The model under review builds one solid part; all positions refer to its coordinate system, in mm. Face numbers are marked on the shaded views. A direction names the side the tool comes from. Round coordinates to 2 decimals unless told otherwise and drop trailing zeros. Loops run counter-clockwise (first coordinate to the right, second up) from the corner with the lowest first, then second, coordinate; pieces in that order, holes last. Notation, with made-up numbers: M 76,-7.5 L 122,-7.5 A25 ccw 122,19.5 Z; hole C -8,-2.5 d9. An arc over 180 degrees is marked long. Answer in a Markdown table with one row per item. Add a question column.
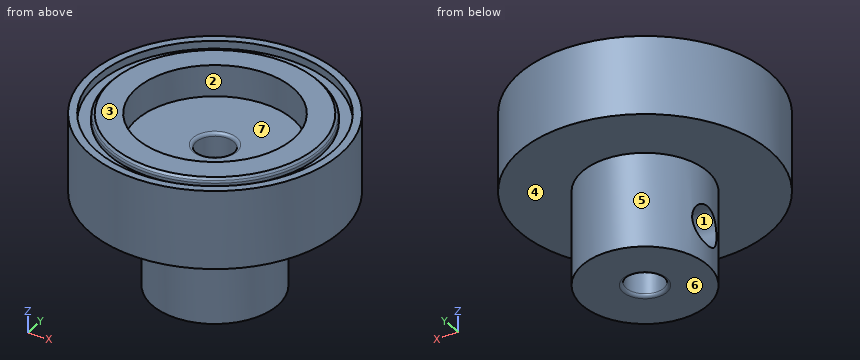
from build123d import *

# Parameters (mm, degrees)
F0_R      = 8
F1_DEPTH  = 5
F2_R      = 4
F3_DEPTH  = 6
F4_R      = 1.2
F5_DEPTH  = 9
F6_R      = 5
F7_DEPTH  = 2
F8_R      = 7.5
F8_R_2    = 6.75
F9_DEPTH  = 0.5
F10_SIZE  = 0.2
F11_R     = 0.2
F13_R     = 1.25
F14_DEPTH = 4.5


with BuildPart() as f1:
    # F0 (on Top) → F1 (new body)
    with BuildSketch(Plane.XY):
        Circle(F0_R)
    extrude(amount=F1_DEPTH)

    # F2 (on face) → F3 (join)
    with BuildSketch(Plane(origin=(0, 0, 0), x_dir=(1, 0, 0), z_dir=(0, 0, -1))):
        Circle(F2_R)
    extrude(amount=F3_DEPTH)

    # F4 (on face) → F5 (cut)
    with BuildSketch(Plane(origin=(0, 0, -6), x_dir=(1, 0, 0), z_dir=(0, 0, -1))):
        Circle(F4_R)
    extrude(amount=-F5_DEPTH, mode=Mode.SUBTRACT)

    # F6 (on face) → F7 (cut)
    with BuildSketch(Plane.XY.offset(5)):
        Circle(F6_R)
    extrude(amount=-F7_DEPTH, mode=Mode.SUBTRACT)

    # F8 (on face) → F9 (cut)
    with BuildSketch(Plane.XY.offset(5)):
        Circle(F8_R)
        Circle(F8_R_2, mode=Mode.SUBTRACT)
    extrude(amount=-F9_DEPTH, mode=Mode.SUBTRACT)

    # F10
    f10_edges = [f1.edges().sort_by_distance(p)[0] for p in [
        (-6.75, 0, 5),
    ]]
    chamfer(f10_edges, length=F10_SIZE)

    # F11
    f11_edges = [f1.edges().sort_by_distance(p)[0] for p in [
        (-6.75, 0, 4.8),
        (-1.2, 0, 3),
        (-1.2, 0, -6),
    ]]
    fillet(f11_edges, radius=F11_R)

    # F13 (on Right) → F14 (cut)
    with BuildSketch(Plane.YZ):
        with Locations((0, -3.5)):
            Circle(F13_R)
    extrude(amount=-F14_DEPTH, mode=Mode.SUBTRACT)


solid = f1.part
1. Machinability: for the marked faces 1, 2, 3 and 4, which of the approach directions +Z, -Z, +X, -X, +Y, -Y give a long, thin tool a straight path to every point of the face, cutting with its end or side? Answer none if there is none.
2. For pin 1 Ø5 at (x, z) = (-4, 4) entering from +Y; pin 2 Ø4.5 at (x, y) = (-2, -1) entering from +Z; pin 3 Ø1 at (y, z) = (5, 3) entering from +X, all flat-tipped, find the tip position at first contact; note any pin that passes through.
3. Take a section at B-B, the plane x = 7.25. State the section outline as (y, z) points.
4. Mouldability with a two-part tool opening along Y and no side actions: class the marked faces 5, 6 and 7 as released by +Y, released by -Y, zero draft, split by the parting line, or undercut.
5. Take a section at A-A, the plane z = -0.25. State the section outline as (x, y) points.
6. Take a section at C-C, the plane y = 0. State how many separate pieces and enclosed holes the cut face has, and give its area (3 significant figures).
7. To check wall thickness, follow probe 1 along Y at (x, z) = (0, 4.6); probe 2 along Y at (x, z) = (0, -2.25); probe 3 along X at (y, z) = (1.25, 4.75). State the ranges of each line that lie inside material, in increasing order.
8. Take a section at D-D, the plane z = -3.5. State the section outline as (x, y) points, and give its area (3 significant figures).
Check sheet entries:
| question | item | result |
|---|---|---|
| 1 | face 1 | -X |
| 1 | face 2 | +Z |
| 1 | face 3 | +Z, +X, -X, +Y, -Y |
| 1 | face 4 | -Z |
| 2 | pin 1 | stops at y = 7.86 |
| 2 | pin 2 | stops at z = 3 |
| 2 | pin 3 | stops at x = 6.61 |
| 3 | outline | M -3.38,0 L 3.38,0 L 3.38,5 L 1.92,5 L 1.92,4.5 L -1.92,4.5 L -1.92,5 L -3.38,5 Z |
| 4 | face 5 | split by the parting line |
| 4 | face 6 | zero draft |
| 4 | face 7 | undercut |
| 5 | outline | C 0,0 d8; hole C 0,0 d2.4 |
| 6 | separate pieces | 3 |
| 6 | enclosed holes | 0 |
| 6 | area | 78.6 mm^2 |
| 7 | probe 1 | y = -8 to -7.5, -6.75 to -5, 5 to 6.75, 7.5 to 8 |
| 7 | probe 2 | y = -4 to -1.2, 1.2 to 4 |
| 7 | probe 3 | x = -7.9 to -7.4, -6.63 to -4.84, 4.84 to 6.63, 7.4 to 7.9 |
| 8 | outline | M -3.8,-1.25 A4 ccw long -3.8,1.25 L 0,1.25 L 0,1.2 A1.2 cw 0,-1.2 L 0,-1.25 Z |
| 8 | area | 38.2 mm^2 |
